The model under review builds one solid part; all positions refer to its coordinate system, in mm. Coordinates: 2 decimals unless noted, no trailing zeros. Write each loop counter-clockwise with the first axis right and the second up, starting at its lowest first coordinate (ties: lowest second). Pieces come first, ordered by that corner, then holes. Notation, with made-up numbers: (7, 61.5) - (55, 61.5) arc R26 ccw to (55, 78.5) - close; hole circle Ø9 at (-35.75, 21). An arc over 180 degrees is marked (long way). Return JSON: item names as keys, results as strings. Group by question number.
(1) We need section C-C on x = -3.5. State the section outline as (y, z) points, then the cut area to 3 significant figures.
(2) For pin 1 Ø1.5 at (x, y) = (19, -6.5) entering from -Z, flat-tipped, find the tip position at first contact; note if it passes through.
(3) We need section D-D on z = 37. State the section outline as (x, y) points.
(4) To check wall thickness, follow L1, parallel to X at y = -0.75, z = 2; L2, parallel to X at y = -3.75, z = 23.5; L3, parallel to X at y = -5, z = 6.5. State the ranges of each line that lie inside material, in increasing order. Write a range as from..to.
(5) We need section A-A on z = 2. State the section outline as (x, y) points.
(6) We need section B-B on y = -6.25. State the section outline as (x, z) points, then the cut area to 3 significant figures.
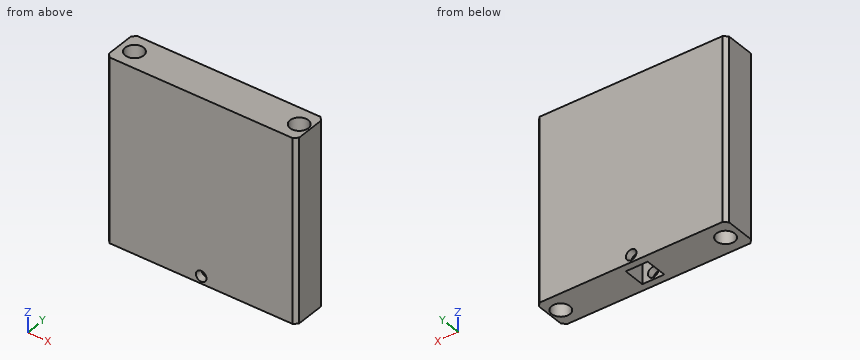
```python
from build123d import *

# Parameters (mm, degrees)
BOSS_EXTRUDE1_DEPTH = 50
SKETCH2_R           = 2.5
CUT_EXTRUDE1_DEPTH  = 68.194635476
SKETCH3_R           = 1.45
CUT_EXTRUDE2_DEPTH  = 68.26652433
SKETCH4_W           = 6
SKETCH4_H           = 6
CUT_EXTRUDE4_DEPTH  = 6


with BuildPart() as part:
    # Sketch1 → Boss-Extrude1 (new body)
    with BuildSketch(Plane.XY):
        Polygon((42.872375084, -9.504406412), (43.872375084, -8.504406412), (43.872375084, -0.504406412), (42.872375084, 0.495593588), (-7.127624916, 0.495593588), (-8.127624916, -0.504406412), (-8.127624916, -8.504406412), (-7.127624916, -9.504406412), align=None)
    extrude(amount=BOSS_EXTRUDE1_DEPTH)

    # Sketch2 → Cut-Extrude1 (cut, through all)
    with BuildSketch(Plane.XY.offset(50)):
        with Locations((-4.127624916, -4.504406412)):
            Circle(SKETCH2_R)
        with Locations((40.872375084, -4.504406412)):
            Circle(SKETCH2_R)
    extrude(amount=-CUT_EXTRUDE1_DEPTH, mode=Mode.SUBTRACT)

    # Sketch3 → Cut-Extrude2 (cut, through all)
    with BuildSketch(Plane.XZ.offset(9.504406412)):
        with Locations(Location((17.872375084, 2, 0), (0, 0, 270))):
            Circle(SKETCH3_R)
    extrude(amount=-CUT_EXTRUDE2_DEPTH, mode=Mode.SUBTRACT)

    # Sketch4 → Cut-Extrude4 (cut)
    with BuildSketch(Plane(origin=(0, 0, 0), x_dir=(-1, 0, 0), z_dir=(0, 0, -1))):
        with Locations((-17.872375084, -4.504406412)):
            Rectangle(SKETCH4_W, SKETCH4_H)
    extrude(amount=-CUT_EXTRUDE4_DEPTH, mode=Mode.SUBTRACT)


solid = part.part
```
Ans:
{
 "1": {"outline": "(-9.5, 0) - (-6.92, 0) - (-6.92, 50) - (-9.5, 50) - close; (-2.08, 0) - (0.5, 0) - (0.5, 50) - (-2.08, 50) - close", "area": "258 mm²"},
 "2": {"pin 1": "z = 6"},
 "3": {"outline": "(-8.13, -8.5) - (-7.13, -9.5) - (42.87, -9.5) - (43.87, -8.5) - (43.87, -0.5) - (42.87, 0.5) - (-7.13, 0.5) - (-8.13, -0.5) - close; hole circle Ø5 at (-4.13, -4.5); hole circle Ø5 at (40.87, -4.5)"},
 "4": {"L1": "-8.13..16.42, 19.32..43.87", "L2": "-8.13..-6.51, -1.74..38.49, 43.26..43.87", "L3": "-8.13..-6.58, -1.68..38.42, 43.32..43.87"},
 "5": {"outline": "(-8.13, -8.5) - (-7.13, -9.5) - (16.42, -9.5) - (16.42, -7.5) - (14.87, -7.5) - (14.87, -1.5) - (16.42, -1.5) - (16.42, 0.5) - (-7.13, 0.5) - (-8.13, -0.5) - close; (19.32, -9.5) - (42.87, -9.5) - (43.87, -8.5) - (43.87, -0.5) - (42.87, 0.5) - (19.32, 0.5) - (19.32, -1.5) - (20.87, -1.5) - (20.87, -7.5) - (19.32, -7.5) - close; hole circle Ø5 at (-4.13, -4.5); hole circle Ø5 at (40.87, -4.5)"},
 "6": {"outline": "(-8.13, 0) - (-5.92, 0) - (-5.92, 50) - (-8.13, 50) - close; (-2.34, 0) - (14.87, 0) - (14.87, 6) - (20.87, 6) - (20.87, 0) - (39.08, 0) - (39.08, 50) - (-2.34, 50) - close; (42.66, 0) - (43.87, 0) - (43.87, 50) - (42.66, 50) - close", "area": "2,210 mm²"}
}
